from build123d import *

# Parameters (mm, degrees)
SCHNITT_LINEAR_AUSTRAGEN1_DEPTH = 2.8
FASE1_SIZE                      = 0.2
VERRUNDUNG1_R                   = 0.2
VERRUNDUNG2_R                   = 0.1


with BuildPart() as part:
    # Skizze1 → Rotation1 (revolve)
    with BuildSketch(Plane(origin=(0, 0, 0), x_dir=(0, 0, -1), z_dir=(1, 0, 0)), mode=Mode.PRIVATE) as rotation1_sk:
        Polygon((-4.9, 0), (-4.9, 4.2), (0, 4.2), (0, 2.45), (25, 2.45), (25, 0), align=None)
    revolve(rotation1_sk.sketch.rotate(Axis((0, 0, 21.919879518), (0, 0, -1)), 90), axis=Axis((0, 0, 21.919879518), (0, 0, -1)))

    # Skizze2 → Schnitt-Linear austragen1 (cut)
    with BuildSketch(Plane.XY.offset(4.9)):
        Polygon((2, -1.154700538), (2, 1.154700538), (0, 2.309401077), (-2, 1.154700538), (-2, -1.154700538), (0, -2.309401077), align=None)
    extrude(amount=-SCHNITT_LINEAR_AUSTRAGEN1_DEPTH, mode=Mode.SUBTRACT)

    # Fase1
    fase1_edges = [part.edges().sort_by_distance(p)[0] for p in [
        (-2.45, 0, -25),
        (-4.2, 0, 0),
        (-4.2, 0, 4.9),
    ]]
    chamfer(fase1_edges, length=FASE1_SIZE)

    # Verrundung1
    verrundung1_edges = [part.edges().sort_by_distance(p)[0] for p in [
        (1, -1.732050808, 2.1),
        (2, -1.154700538, 3.5),
        (-1, -1.732050808, 2.1),
        (0, -2.309401077, 3.5),
        (-2, 0, 2.1),
        (-2, -1.154700538, 3.5),
        (-1, 1.732050808, 2.1),
        (-2, 1.154700538, 3.5),
        (1, 1.732050808, 2.1),
        (0, 2.309401077, 3.5),
        (2, 0, 2.1),
        (2, 1.154700538, 3.5),
        (-2.45, 0, 0),
    ]]
    fillet(verrundung1_edges, radius=VERRUNDUNG1_R)

    # Verrundung2
    verrundung2_edges = [part.edges().sort_by_distance(p)[0] for p in [
        (-1, -1.732050808, 4.9),
        (-2, 0, 4.9),
        (-1, 1.732050808, 4.9),
        (1, 1.732050808, 4.9),
        (2, 0, 4.9),
        (1, -1.732050808, 4.9),
        (-1.973205081, -1.139230485, 4.9),
        (0, -2.278460969, 4.9),
        (1.973205081, -1.139230485, 4.9),
        (1.973205081, 1.139230485, 4.9),
        (0, 2.278460969, 4.9),
        (-1.973205081, 1.139230485, 4.9),
    ]]
    fillet(verrundung2_edges, radius=VERRUNDUNG2_R)


solid = part.part
For this review, take the finished solid that the model builds, in its own axes (mm). A direction names the side the tool comes from. Give positions to 0.01 mm unless a question says otherwise; leave off trailing zeros. Order: outer loops, then holes, each group sorted by start corner. A loop starts at its lowest first (then second) coordinate and runs counter-clockwise, first axis right, second up. Notation, with made-up numbers: M 76.5,-5 L 86.5,-5 A27 cw 86.5,13 Z; hole C 9,15.25 d5. An arc over 180 degrees is marked long. Answer in a Markdown table with one row per item. Add a question column.
(1) Wall thickness on probe 1 along Z at (x, y) = (1.5, 3.25); probe 2 along Y at (x, z) = (-1.25, -11.5); probe 3 along Y at (x, z) = (0.5, 2.75): over which ranges is each line inside the solid? List them lowest first. Write a range as [from, to].
(2) Consider section B-B on z = -19. State the section outline as (x, y) points, and give its area (3 significant figures).
(3) For faces 1 (the face through (0, 0, -25)), 2 (the face through (0.99, -1.74, 3.57)), list the 3-axis set-ups (+Z, -Z, +X, -X, +Y, -Y) from which the entire face can be reached by the end or side of a thin tool; tool diameter is ignored.
(4) For pin 1 (1 mm diameter, centred on x = -2, z = -20, fed in from +Y); pin 2 (0.6 mm diameter, centred on y = -0.5, z = 4, fed in from +X); pin 3 (5 mm diameter, centred on y = -0.5, z = -8, fed in from -X), all flat-tipped, find the tip position at first contact; note any pin that passes through.
(5) Mouldability with a two-part tool opening along Y and no side actions: class faces 3 (the face through (-1.013, -1.725, 3.568)), 4 (the face through (-2, 0, 4)), 5 (the face through (-2, 2, 4.9)), 6 (the face through (-1.806, -1.656, -12.672)) as +Y half, -Y half, draft (parallel to the pull), parting line (faces both ways), or undercut.
(6) Consider section A-A on y = 0. State the section outline as (x, z) points.
Evaluation:
| question | item | result |
|---|---|---|
| 1 | probe 1 | z = [0, 4.9] |
| 1 | probe 2 | y = [-2.11, 2.11] |
| 1 | probe 3 | y = [-4.17, -2.02], [2.02, 4.17] |
| 2 | outline | C 0,0 d4.9 |
| 2 | area | 18.9 mm^2 |
| 3 | face 1 | -Z, +X, -X, +Y, -Y |
| 3 | face 2 | +Z |
| 4 | pin 1 | stops at y = 1.94 |
| 4 | pin 2 | stops at x = 4.2 |
| 4 | pin 3 | stops at x = -2.45 |
| 5 | face 3 | undercut |
| 5 | face 4 | undercut |
| 5 | face 5 | draft |
| 5 | face 6 | parting line |
| 6 | outline | M -4.2,0.2 L -4,0 L -2.65,0 A0.2 cw -2.45,-0.2 L -2.45,-24.8 L -2.25,-25 L 2.25,-25 L 2.45,-24.8 L 2.45,-0.2 A0.2 cw 2.65,0 L 4,0 L 4.2,0.2 L 4.2,4.7 L 4,4.9 L 2.1,4.9 A0.1 ccw 2,4.8 L 2,2.3 A0.2 cw 1.8,2.1 L -1.8,2.1 A0.2 cw -2,2.3 L -2,4.8 A0.1 ccw -2.1,4.9 L -4,4.9 L -4.2,4.7 Z |
